```python
from build123d import *

# Parameters (mm, degrees)
SKETCH1_W           = 89.5
SKETCH1_H           = 50.8
BOSS_EXTRUDE1_DEPTH = 1.5875
CHAMFER1_SIZE       = 2
CUT_EXTRUDE1_DEPTH  = 2.5875
SKETCH3_R           = 1.75
CUT_EXTRUDE2_DEPTH  = 2.5875
CHAMFER2_SIZE       = 1.27


with BuildPart() as part:
    # Sketch1 → Boss-Extrude1 (new body)
    with BuildSketch(Plane.XY):
        with Locations((44.75, 25.4)):
            Rectangle(SKETCH1_W, SKETCH1_H)
    extrude(amount=BOSS_EXTRUDE1_DEPTH)

    # Chamfer1
    chamfer1_edges = [part.edges().sort_by_distance(p)[0] for p in [
        (0, 50.8, 0.79375),
        (89.5, 50.8, 0.79375),
        (89.5, 0, 0.79375),
        (0, 0, 0.79375),
    ]]
    chamfer(chamfer1_edges, length=CHAMFER1_SIZE)

    # Sketch2 → Cut-Extrude1 (cut, through all)
    with BuildSketch(Plane(origin=(0, 0, 0), x_dir=(-1, 0, 0), z_dir=(0, 0, -1))):
        with BuildLine():
            Line((-43.559375, 41.275), (-43.559375, 9.525))
            ThreePointArc((-43.559375, 9.525), (-44.75, 8.334375), (-45.940625, 9.525))
            Line((-45.940625, 9.525), (-45.940625, 41.275))
            ThreePointArc((-45.940625, 41.275), (-44.75, 42.465625), (-43.559375, 41.275))
        make_face()
        with BuildLine():
            Line((-38.479375, 41.275), (-38.479375, 9.525))
            ThreePointArc((-38.479375, 9.525), (-39.67, 8.334375), (-40.860625, 9.525))
            Line((-40.860625, 9.525), (-40.860625, 41.275))
            ThreePointArc((-40.860625, 41.275), (-39.67, 42.465625), (-38.479375, 41.275))
        make_face()
        with BuildLine():
            Line((-33.399375, 41.275), (-33.399375, 9.525))
            ThreePointArc((-33.399375, 9.525), (-34.59, 8.334375), (-35.780625, 9.525))
            Line((-35.780625, 9.525), (-35.780625, 41.275))
            ThreePointArc((-35.780625, 41.275), (-34.59, 42.465625), (-33.399375, 41.275))
        make_face()
        with BuildLine():
            Line((-28.319375, 41.275), (-28.319375, 9.525))
            ThreePointArc((-28.319375, 9.525), (-29.51, 8.334375), (-30.700625, 9.525))
            Line((-30.700625, 9.525), (-30.700625, 41.275))
            ThreePointArc((-30.700625, 41.275), (-29.51, 42.465625), (-28.319375, 41.275))
        make_face()
        with BuildLine():
            Line((-23.239375, 41.275), (-23.239375, 9.525))
            ThreePointArc((-23.239375, 9.525), (-24.43, 8.334375), (-25.620625, 9.525))
            Line((-25.620625, 9.525), (-25.620625, 41.275))
            ThreePointArc((-25.620625, 41.275), (-24.43, 42.465625), (-23.239375, 41.275))
        make_face()
        with BuildLine():
            Line((-18.159375, 41.275), (-18.159375, 9.525))
            ThreePointArc((-18.159375, 9.525), (-19.35, 8.334375), (-20.540625, 9.525))
            Line((-20.540625, 9.525), (-20.540625, 41.275))
            ThreePointArc((-20.540625, 41.275), (-19.35, 42.465625), (-18.159375, 41.275))
        make_face()
        with BuildLine():
            Line((-13.079375, 41.275), (-13.079375, 9.525))
            ThreePointArc((-13.079375, 9.525), (-14.27, 8.334375), (-15.460625, 9.525))
            Line((-15.460625, 9.525), (-15.460625, 41.275))
            ThreePointArc((-15.460625, 41.275), (-14.27, 42.465625), (-13.079375, 41.275))
        make_face()
        with BuildLine():
            Line((-7.999375, 41.275), (-7.999375, 9.525))
            ThreePointArc((-7.999375, 9.525), (-9.19, 8.334375), (-10.380625, 9.525))
            Line((-10.380625, 9.525), (-10.380625, 41.275))
            ThreePointArc((-10.380625, 41.275), (-9.19, 42.465625), (-7.999375, 41.275))
        make_face()
        with BuildLine():
            Line((-2.919375, 41.275), (-2.919375, 9.525))
            ThreePointArc((-2.919375, 9.525), (-4.11, 8.334375), (-5.300625, 9.525))
            Line((-5.300625, 9.525), (-5.300625, 41.275))
            ThreePointArc((-5.300625, 41.275), (-4.11, 42.465625), (-2.919375, 41.275))
        make_face()
        with BuildLine():
            Line((-48.639375, 41.275), (-48.639375, 9.525))
            ThreePointArc((-48.639375, 9.525), (-49.83, 8.334375), (-51.020625, 9.525))
            Line((-51.020625, 9.525), (-51.020625, 41.275))
            ThreePointArc((-51.020625, 41.275), (-49.83, 42.465625), (-48.639375, 41.275))
        make_face()
        with BuildLine():
            Line((-53.719375, 41.275), (-53.719375, 9.525))
            ThreePointArc((-53.719375, 9.525), (-54.91, 8.334375), (-56.100625, 9.525))
            Line((-56.100625, 9.525), (-56.100625, 41.275))
            ThreePointArc((-56.100625, 41.275), (-54.91, 42.465625), (-53.719375, 41.275))
        make_face()
        with BuildLine():
            Line((-58.799375, 41.275), (-58.799375, 9.525))
            ThreePointArc((-58.799375, 9.525), (-59.99, 8.334375), (-61.180625, 9.525))
            Line((-61.180625, 9.525), (-61.180625, 41.275))
            ThreePointArc((-61.180625, 41.275), (-59.99, 42.465625), (-58.799375, 41.275))
        make_face()
        with BuildLine():
            Line((-63.879375, 41.275), (-63.879375, 9.525))
            ThreePointArc((-63.879375, 9.525), (-65.07, 8.334375), (-66.260625, 9.525))
            Line((-66.260625, 9.525), (-66.260625, 41.275))
            ThreePointArc((-66.260625, 41.275), (-65.07, 42.465625), (-63.879375, 41.275))
        make_face()
        with BuildLine():
            Line((-68.959375, 41.275), (-68.959375, 9.525))
            ThreePointArc((-68.959375, 9.525), (-70.15, 8.334375), (-71.340625, 9.525))
            Line((-71.340625, 9.525), (-71.340625, 41.275))
            ThreePointArc((-71.340625, 41.275), (-70.15, 42.465625), (-68.959375, 41.275))
        make_face()
        with BuildLine():
            Line((-74.039375, 41.275), (-74.039375, 9.525))
            ThreePointArc((-74.039375, 9.525), (-75.23, 8.334375), (-76.420625, 9.525))
            Line((-76.420625, 9.525), (-76.420625, 41.275))
            ThreePointArc((-76.420625, 41.275), (-75.23, 42.465625), (-74.039375, 41.275))
        make_face()
        with BuildLine():
            Line((-79.119375, 41.275), (-79.119375, 9.525))
            ThreePointArc((-79.119375, 9.525), (-80.31, 8.334375), (-81.500625, 9.525))
            Line((-81.500625, 9.525), (-81.500625, 41.275))
            ThreePointArc((-81.500625, 41.275), (-80.31, 42.465625), (-79.119375, 41.275))
        make_face()
        with BuildLine():
            Line((-84.199375, 41.275), (-84.199375, 9.525))
            ThreePointArc((-84.199375, 9.525), (-85.39, 8.334375), (-86.580625, 9.525))
            Line((-86.580625, 9.525), (-86.580625, 41.275))
            ThreePointArc((-86.580625, 41.275), (-85.39, 42.465625), (-84.199375, 41.275))
        make_face()
    extrude(amount=-CUT_EXTRUDE1_DEPTH, mode=Mode.SUBTRACT)

    # Sketch3 → Cut-Extrude2 (cut, through all)
    with BuildSketch(Plane(origin=(0, 0, 0), x_dir=(-1, 0, 0), z_dir=(0, 0, -1))):
        with Locations((-85.75, 47.15)):
            Circle(SKETCH3_R)
        with Locations((-3.75, 47.15)):
            Circle(SKETCH3_R)
        with Locations((-3.75, 3.65)):
            Circle(SKETCH3_R)
        with Locations((-85.75, 3.65)):
            Circle(SKETCH3_R)
    extrude(amount=-CUT_EXTRUDE2_DEPTH, mode=Mode.SUBTRACT)

    # Chamfer2
    chamfer2_edges = [part.edges().sort_by_distance(p)[0] for p in [
        (87.5, 47.15, 0),
        (5.5, 47.15, 0),
        (5.5, 3.65, 0),
        (87.5, 3.65, 0),
    ]]
    chamfer(chamfer2_edges, length=CHAMFER2_SIZE)


solid = part.part
```
Build history of the part. All positions in model axes, mm. Give positions to 0.01 mm unless a question says otherwise; leave off trailing zeros. Loops run counter-clockwise (first coordinate to the right, second up) from the corner with the lowest first, then second, coordinate; pieces in that order, holes last.
1) Drop a flat-ended pin along its axis: P1, Ø3, axis at x = 85.75, y = 3.65, coming from the +Z side. Give the stop position or say it passes through.
Values follow:
P1: passes through
2) Probe line 1 along Y through (x, z) = (70, 0.45); line 2 along Y through (x, z) = (3.75, 1.5); line 3 along Y through (x, z) = (81, 1.2). List the from-to ranges inside material, lowest first.
Values follow:
line 1: y = 0 to 8.34, 42.46 to 50.8
line 2: y = 0 to 1.9, 5.4 to 8.39, 42.41 to 45.4, 48.9 to 50.8
line 3: y = 0 to 8.55, 42.25 to 50.8
3) Band-saw the part on A-A on x = 65.07. List the corners of the cut face in (y, z).
Values follow:
outline: (0, 0) - (8.33, 0) - (8.33, 1.59) - (0, 1.59) - close; (42.47, 0) - (50.8, 0) - (50.8, 1.59) - (42.47, 1.59) - close
4) Band-saw the part on B-B on z = 1. State how many separate pieces and enclosed holes the cut face has, then the cut area to 3 significant figures.
Values follow:
separate pieces: 1
enclosed holes: 21
area: 3,130 mm2
5) Two-plate mould, pull along X, no slides. Class faces 1 (the face through (56.101, 25, 1)), 2 (the face through (9.164, 8.335, 0.783)), 3 (the face through (1, 1, 1)): released by +X, released by -X, zero draft, split by the parting line, or undercut.
Values follow:
face 1: undercut
face 2: undercut
face 3: released by -X
